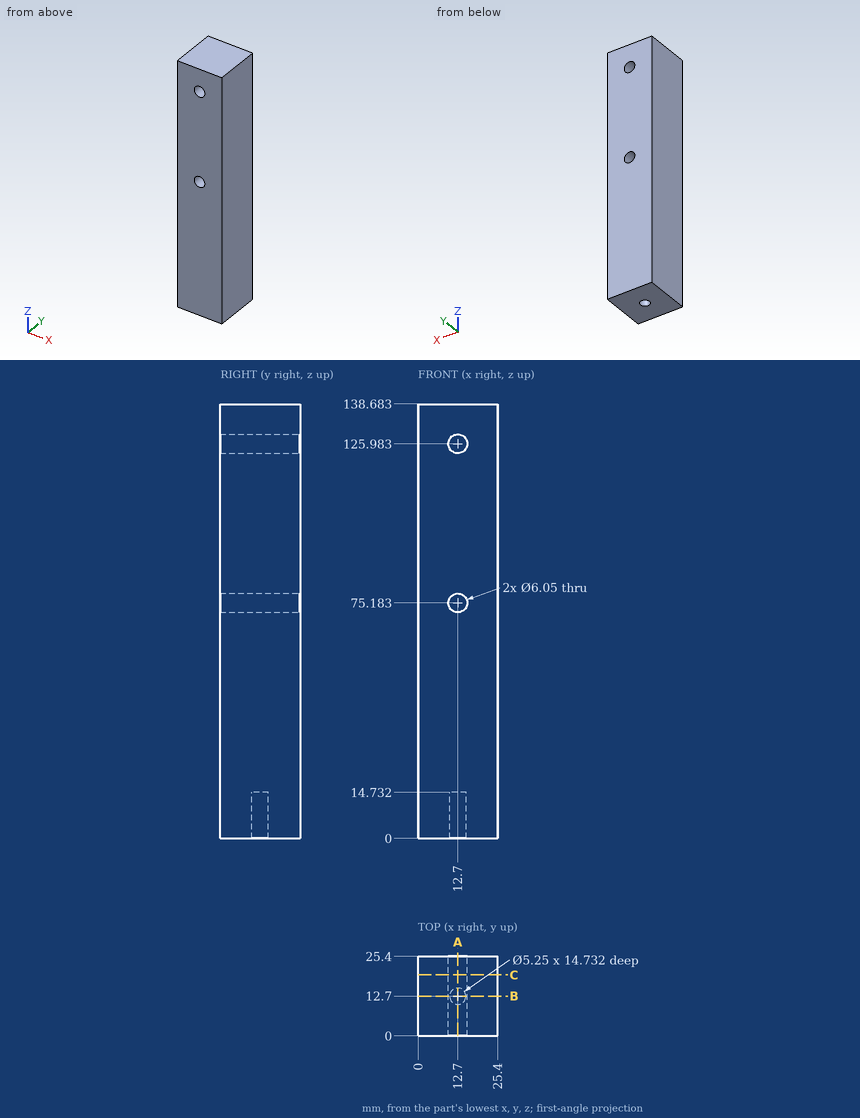
For this review, use the dimensioned drawing (mm, ordinates from the lowest corner) and the shaded views. Coordinates: 2 decimals unless noted, no trailing zeros. Loops run counter-clockwise (first coordinate to the right, second up) from the corner with the lowest first, then second, coordinate; pieces in that order, holes last. Notation, with made-up numbers: (51.5, 77.25) - (102.5, 77.25) arc R13 cw to (102.5, 90.25) - close; hole circle Ø3 at (43, 9.25). An arc over 180 degrees is marked (long way). Use CSV: the item, a comma, the result in double quotes. Start each with the question number.
1) Consider section A-A on x = 12.7. Write out the cut boundary in (y, z) (3 decimals).
2) Consider section C-C on y = 19.5. Write out the cut boundary in (x, z) (3 decimals), then the cut area to 3 significant figures.
3) Wall thickness on L1, parallel to Z at x = 12.7, y = 10.5; L2, parallel to Z at x = 12.7, y = 18.5; L3, parallel to X at y = 13, z = 127.5: over which ranges is each line inside the solid? List them lowest first. Write a range as from..to.
4) Consider section B-B on y = 12.7. Write out the cut boundary in (x, z) (3 decimals).
Geometry says:
1,outline,"(0, 0) - (10.075, 0) - (10.075, 14.732) - (15.325, 14.732) - (15.325, 0) - (25.4, 0) - (25.4, 72.158) - (0, 72.158) - close; (0, 78.208) - (25.4, 78.208) - (25.4, 122.958) - (0, 122.958) - close; (0, 129.008) - (25.4, 129.008) - (25.4, 138.683) - (0, 138.683) - close"
2,outline,"(0, 0) - (25.4, 0) - (25.4, 138.683) - (0, 138.683) - close; hole circle Ø6.05 at (12.7, 75.183); hole circle Ø6.05 at (12.7, 125.983)"
2,area,"3,470 mm^2"
3,L1,"14.73..72.16, 78.21..122.96, 129.01..138.68"
3,L2,"0..72.16, 78.21..122.96, 129.01..138.68"
3,L3,"0..10.08, 15.32..25.4"
4,outline,"(0, 0) - (10.075, 0) - (10.075, 14.732) - (15.325, 14.732) - (15.325, 0) - (25.4, 0) - (25.4, 138.683) - (0, 138.683) - close; hole circle Ø6.05 at (12.7, 75.183); hole circle Ø6.05 at (12.7, 125.983)"
